Geometry: final body of the model. Coordinates: model frame, mm. A direction names the side the tool comes from. Coordinates: 2 decimals unless noted, no trailing zeros. Write each loop counter-clockwise with the first axis right and the second up, starting at its lowest first coordinate (ties: lowest second). Pieces come first, ordered by that corner, then holes.
from build123d import *

# Parameters (mm, degrees)
SKETCH1_R           = 7
SKETCH1_R_2         = 4
BOSS_EXTRUDE1_DEPTH = 10
SKETCH2_R           = 1.5
CUT_EXTRUDE1_DEPTH  = 10


with BuildPart() as part:
    # Sketch1 → Boss-Extrude1 (new body)
    with BuildSketch(Plane(origin=(0, 0, 0), x_dir=(1, 0, 0), z_dir=(0, 1, 0))):
        with BuildLine():
            Line((-1.7425, -20.4258095), (-101.02, -11.956571415))
            ThreePointArc((-101.02, -11.956571415), (-112, 0), (-101.02, 11.956571415))
            Line((-101.02, 11.956571415), (-1.7425, 20.4258095))
            ThreePointArc((-1.7425, 20.4258095), (20.5, 0), (-1.7425, -20.4258095))
        make_face()
        with Locations(Location((0, 0, 0), (0, 0, 270))):
            Circle(SKETCH1_R, mode=Mode.SUBTRACT)
        with Locations(Location((-100, 0, 0), (0, 0, 270))):
            Circle(SKETCH1_R_2, mode=Mode.SUBTRACT)
        with BuildLine():
            Line((-84.191001334, -3.779047898), (-81.096242799, -2.881194367))
            ThreePointArc((-81.096242799, -2.881194367), (-78.932136943, 0), (-81.096242799, 2.881194367))
            Line((-81.096242799, 2.881194367), (-84.191001334, 3.779047898))
            ThreePointArc((-84.191001334, 3.779047898), (-86.899619701, 3.241548046), (-88.021516382, 0.718282824))
            ThreePointArc((-88.021516382, 0.718282824), (-88, 0), (-88.021516382, -0.718282824))
            ThreePointArc((-88.021516382, -0.718282824), (-86.899619701, -3.241548046), (-84.191001334, -3.779047898))
        make_face(mode=Mode.SUBTRACT)
        with BuildLine():
            Line((-69.832249651, -3.778216146), (-65.93770065, -2.648326841))
            ThreePointArc((-65.93770065, -2.648326841), (-63.987280982, -2.371113698), (-62.036861314, -2.648326841))
            Line((-62.036861314, -2.648326841), (-53.969530614, -4.988826518))
            ThreePointArc((-53.969530614, -4.988826518), (-51.855920685, -8.418131938), (-55.060424757, -10.859163739))
            Line((-55.060424757, -10.859163739), (-69.251355507, -9.648553367))
            ThreePointArc((-69.251355507, -9.648553367), (-71.98177462, -6.95483008), (-69.832249651, -3.778216146))
        make_face(mode=Mode.SUBTRACT)
        with BuildLine():
            Line((-46.878319164, -2.881194367), (-23.320026626, -9.715942825))
            ThreePointArc((-23.320026626, -9.715942825), (-20.349346369, -8.942517006), (-19.613817698, -5.962227378))
            ThreePointArc((-19.613817698, -5.962227378), (-20.5, 0), (-19.613817698, 5.962227378))
            ThreePointArc((-19.613817698, 5.962227378), (-20.349346369, 8.942517006), (-23.320026626, 9.715942825))
            Line((-23.320026626, 9.715942825), (-46.878319164, 2.881194367))
            ThreePointArc((-46.878319164, 2.881194367), (-49.042425021, 0), (-46.878319164, -2.881194367))
        make_face(mode=Mode.SUBTRACT)
        with BuildLine():
            Line((-62.036861314, 2.648326841), (-53.969530614, 4.988826518))
            ThreePointArc((-53.969530614, 4.988826518), (-51.855920685, 8.418131938), (-55.060424757, 10.859163739))
            Line((-55.060424757, 10.859163739), (-69.251355507, 9.648553367))
            ThreePointArc((-69.251355507, 9.648553367), (-71.98177462, 6.95483008), (-69.832249651, 3.778216146))
            Line((-69.832249651, 3.778216146), (-65.93770065, 2.648326841))
            ThreePointArc((-65.93770065, 2.648326841), (-63.987280982, 2.371113698), (-62.036861314, 2.648326841))
        make_face(mode=Mode.SUBTRACT)
    extrude(amount=BOSS_EXTRUDE1_DEPTH)

    # Sketch2 → Cut-Extrude1 (cut)
    with BuildSketch(Plane(origin=(0, 10, 0), x_dir=(1, 0, 0), z_dir=(0, 1, 0))):
        with Locations(Location((-15.5, 0, 0), (0, 0, 270))):
            Circle(SKETCH2_R)
        with Locations(Location((0, 15.5, 0), (0, 0, 270))):
            Circle(SKETCH2_R)
        with Locations(Location((15.5, 0, 0), (0, 0, 270))):
            Circle(SKETCH2_R)
        with Locations(Location((0, -15.5, 0), (0, 0, 270))):
            Circle(SKETCH2_R)
    extrude(amount=-CUT_EXTRUDE1_DEPTH, mode=Mode.SUBTRACT)


solid = part.part
Item 1: Section B-B, the plane y = 6.25. State how many separate pieces and enclosed holes the cut face has, plus the area to 3 significant figures.
Derived:
separate pieces: 1
enclosed holes: 10
area: 3,230 mm2
Item 2: Section C-C, the plane z = 15.5. Output: boundary loops of the cut face in (x, y).
Derived:
outline: (-59.48, 0) - (-1.5, 0) - (-1.5, 10) - (-59.48, 10) - close; (1.5, 0) - (13.42, 0) - (13.42, 10) - (1.5, 10) - close
Item 3: Pin query (flat end, axial travel): pin 1 (1 mm diameter, centred on y = 6.5, z = 3, fed in from +X); pin 2 (1.5 mm diameter, centred on x = -67, y = 5, fed in from +Z). Return the tip coordinate at first contact, or that it passes through.
Derived:
pin 1: stops at x = 20.35
pin 2: stops at z = 14.92
Item 4: Material intervals for probe 1 along Z at (x, y) = (-2.5, 8.5); probe 2 along Z at (x, y) = (-39.5, 6.5); probe 3 along Z at (x, y) = (-53, 5.75), sorted ascending.
Derived:
probe 1: z = -20.36 to -6.54, 6.54 to 20.36
probe 2: z = -17.2 to -5.02, 5.02 to 17.2
probe 3: z = -16.05 to -10.27, -5.47 to 5.47, 10.27 to 16.05
Item 5: Section A-A, the plane x = 0. Output: boundary loops of the cut face in (y, z), plus the area to 3 significant figures.
Derived:
outline: (0, -20.5) - (10, -20.5) - (10, -17) - (0, -17) - close; (0, -14) - (10, -14) - (10, -7) - (0, -7) - close; (0, 7) - (10, 7) - (10, 14) - (0, 14) - close; (0, 17) - (10, 17) - (10, 20.5) - (0, 20.5) - close
area: 210 mm2
Item 6: Section D-D, the plane x = -15.5. Output: boundary loops of the cut face in (y, z), plus the area to 3 significant figures.
Derived:
outline: (0, -19.25) - (10, -19.25) - (10, -1.5) - (0, -1.5) - close; (0, 1.5) - (10, 1.5) - (10, 19.25) - (0, 19.25) - close
area: 355 mm2
Item 7: Pull-direction query (Z, two-part tool) for faces 1 (the flat face through (-50.69, 4.93, 16.25)), 2 (the cylindrical face through (-51.845, 4.93, -8.357)), 3 (the cylindrical face through (-112, 5, 0)); classes: released by +Z, released by -Z, zero draft, split by the parting line, or undercut.
Derived:
face 1: released by +Z
face 2: undercut
face 3: split by the parting line
Item 8: Set-up query: faces 4 (the flat face through (-45, 10, 4)), 5 (the flat face through (-82.622, 4.93, -3.324)). Return all of +Z, -Z, +X, -X, +Y, -Y with unobstructed straight access to the full face (end or side cutting, diameter ignored); none if empty.
Derived:
face 4: +Z, -Z, +X, -X, +Y
face 5: +Y, -Y
